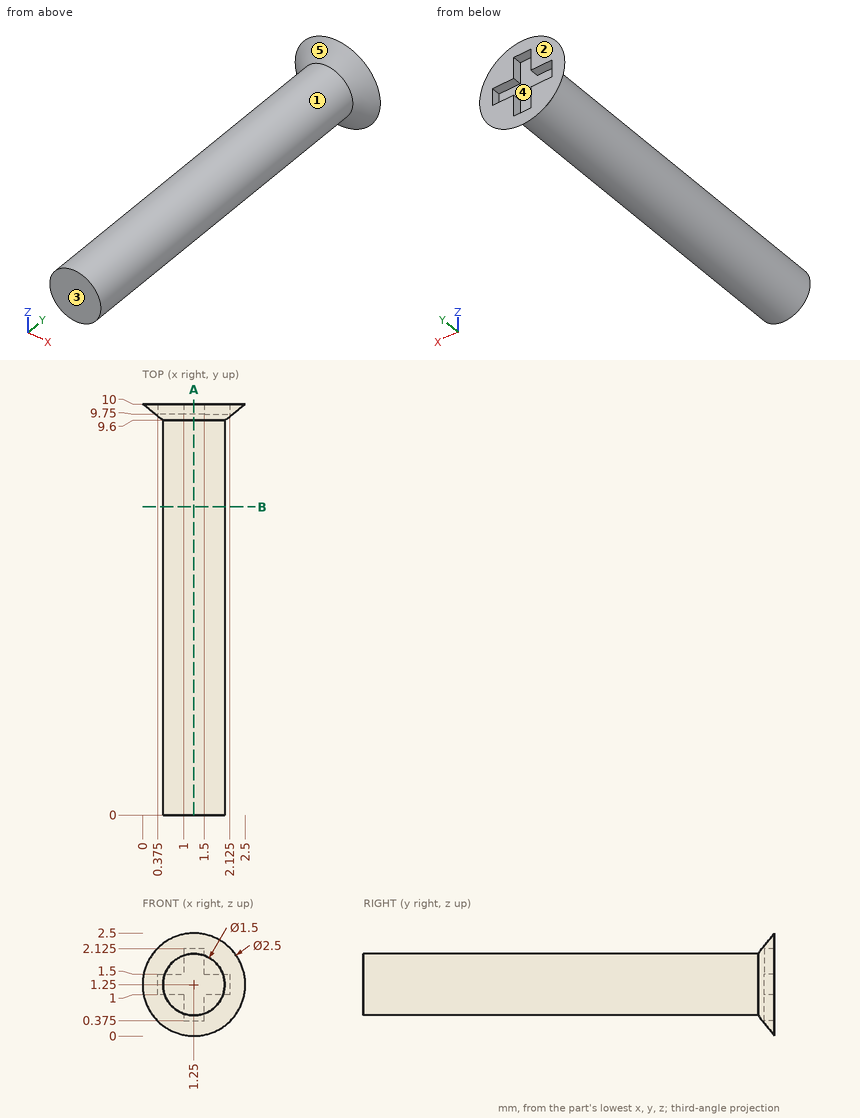
Part print with two shaded views. Sizes in mm from the minimum x, y, z corner. A direction names the side the tool comes from. Round coordinates to 2 decimals unless told otherwise and drop trailing zeros. Write each loop counter-clockwise with the first axis right and the second up, starting at its lowest first coordinate (ties: lowest second). Pieces come first, ordered by that corner, then holes. Notation, with made-up numbers: M 59.5,53.5 L 67.5,53.5 A25 cw 67.5,78.5 Z; hole C 28.5,44.25 d6. An arc over 180 degrees is marked long. Put each result on its own line as item: value. Start each with the question number.
1) Drill centre lines: probe 1 along Y at (x, z) = (1.3, 0.95); probe 2 along X at (y, z) = (8.5, 1.2); probe 3 along X at (y, z) = (3.5, 0.8). Where is each one in solid material? Low to high. Write a range as [from, to].
2) Saw through at A-A, the plane x = 1.25. Write the cut outline in (y, z) (3 decimals).
3) 3-axis set-ups, long thin cutter, end or side, ignore diameter. For the marked faces 1 and 2: which of +Z, -Z, +X, -X, +Y, -Y reach the whole face in a straight line?
4) Saw through at B-B, the plane y = 7.5. Write the cut outline in (x, z).
5) Pull direction Z, two halves, no side cores. Call the marked faces 3, 4 and 5: pulls with the +Z half, pulls with the -Z half, needs draft (parallel to the pull), parting line crosses it, or undercut.
6) Pin check, flat tip, straight feed: pin 1 Ø1 at (x, y) = (1.5, 6.5) entering from +Z. Stop position of the tip, or through.
Resolved:
1. probe 1: [0, 9.75]
1. probe 2: [0.5, 2]
1. probe 3: [0.65, 1.85]
2. outline: M 0,0.5 L 9.6,0.5 L 10,0 L 10,0.375 L 9.75,0.375 L 9.75,2.125 L 10,2.125 L 10,2.5 L 9.6,2 L 0,2 Z
3. face 1: -Y
3. face 2: +Z, -Z, +X, -X, +Y
4. outline: C 1.25,1.25 d1.5
5. face 3: needs draft
5. face 4: undercut
5. face 5: parting line crosses it
6. pin 1: z = 2
